from build123d import *

# Parameters (mm, degrees)
SKETCH_2_R          = 1.9
CUT_EXTRUDE_1_DEPTH = 36


with BuildPart() as part:
    # 草图1 → 旋转1 (revolve)
    with BuildSketch(Plane(origin=(0, 0, 0), x_dir=(1, 0, 0), z_dir=(0, 1, 0)), mode=Mode.PRIVATE) as revolve_1_sk:
        Polygon((0, -1e-09), (0, -35), (6, -35), (6, -30), (7.5, -30), (7.5, -26), (9, -26), (13, -26), (13, -9), (9, -9), (7.5, -9), (7.5, -5), (6, -5), (6, -1e-09), align=None)
    revolve(revolve_1_sk.sketch.rotate(Axis((0, 0, 1e-09), (0, 0, 1)), 180), axis=Axis((0, 0, 1e-09), (0, 0, 1)))

    # 草图2 → 切除-拉伸1 (cut)
    with BuildSketch(Plane.XY.offset(35)):
        Circle(SKETCH_2_R)
    extrude(amount=-CUT_EXTRUDE_1_DEPTH, mode=Mode.SUBTRACT)


solid = part.part
For this review, take the finished solid that the model builds, in its own axes (mm). A direction names the side the tool comes from. Give positions to 0.01 mm unless a question says otherwise; leave off trailing zeros. Order: outer loops, then holes, each group sorted by start corner. A loop starts at its lowest first (then second) coordinate and runs counter-clockwise, first axis right, second up. Notation, with made-up numbers: (-2, -2.5) - (57, -2.5) arc R33 ccw to (57, 26.5) - close; hole circle Ø6 at (23.25, 83). An arc over 180 degrees is marked (long way). Answer as a JSON object with one key per item and string values. Group by question number.
Item 1: Machinability: for faces 1 (the cylindrical face through (-4.032, -6.324, 6.972)), 2 (the flat face through (3, 0, 35)), 3 (the flat face through (6, 6, 26)), which of the approach directions +Z, -Z, +X, -X, +Y, -Y give a long, thin tool a straight path to every point of the face, cutting with its end or side? Answer none if there is none.
Item 2: Take a section at C-C on z = 31. Give the boundary of the cut face in (x, y), and give its area (3 significant figures).
Item 3: Take a section at A-A on x = 0. Give the boundary of the cut face in (y, z), and give its area (3 significant figures).
Item 4: Wall thickness on line 1 along Y through (x, z) = (0, 27.5); line 2 along Y through (x, z) = (0, 12.5); line 3 along Z through (x, y) = (-2.5, -8): over which ranges is each line inside the solid? List them lowest first.
Item 5: Take a section at D-D on x = 3.5. Give the boundary of the cut face in (y, z), and give its area (3 significant figures).
Item 6: Draft analysis for pull direction X (two halves, no side actions). For faces 4 (the cylindrical face through (-1.9, 0.08, 17.75)), 5 (the flat face through (-3, 0, 0)), 6 (the cylindrical face through (-5.723, -1.802, 32.465)), state which applies: pulls with the +X half, pulls with the -X half, needs draft (parallel to the pull), parting line crosses it, or undercut.
Item 7: Clearance check with a flat-ended pin moving along its axis: pin 1 Ø4.5 at (x, y) = (-0.5, 1.5) entering from +Z. State where the tip first meets the part, or that it passes through.
Reported:
{
 "1": {"face 1": "-Z", "face 2": "+Z, +X, -X, +Y, -Y", "face 3": "+Z"},
 "2": {"outline": "circle Ø12 at (0, 0); hole circle Ø3.8 at (0, 0)", "area": "102 mm^2"},
 "3": {"outline": "(-13, 9) - (-7.5, 9) - (-7.5, 5) - (-6, 5) - (-6, 0) - (-1.9, 0) - (-1.9, 35) - (-6, 35) - (-6, 30) - (-7.5, 30) - (-7.5, 26) - (-13, 26) - close; (1.9, 0) - (6, 0) - (6, 5) - (7.5, 5) - (7.5, 9) - (13, 9) - (13, 26) - (7.5, 26) - (7.5, 30) - (6, 30) - (6, 35) - (1.9, 35) - close", "area": "549 mm^2"},
 "4": {"line 1": "-7.5 to -1.9, 1.9 to 7.5", "line 2": "-13 to -1.9, 1.9 to 13", "line 3": "9 to 26"},
 "5": {"outline": "(-12.52, 9) - (-6.63, 9) - (-6.63, 5) - (-4.87, 5) - (-4.87, 0) - (4.87, 0) - (4.87, 5) - (6.63, 5) - (6.63, 9) - (12.52, 9) - (12.52, 26) - (6.63, 26) - (6.63, 30) - (4.87, 30) - (4.87, 35) - (-4.87, 35) - (-4.87, 30) - (-6.63, 30) - (-6.63, 26) - (-12.52, 26) - close", "area": "629 mm^2"},
 "6": {"face 4": "undercut", "face 5": "needs draft", "face 6": "parting line crosses it"},
 "7": {"pin 1": "z = 35"}
}
